Source: CAD feature listing. Evaluate the final solid. Frame: model axes, mm. Face numbers are marked on the shaded views. A direction names the side the tool comes from. Coordinates: 2 decimals unless noted, no trailing zeros. Write each loop counter-clockwise with the first axis right and the second up, starting at its lowest first coordinate (ties: lowest second). Pieces come first, ordered by that corner, then holes. Notation, with made-up numbers: M 21,-23.75 L 51,-23.75 A26 cw 51,8.25 Z; hole C 26.5,1.5 d2. An arc over 180 degrees is marked long. Write item = value, one per line. Start each with the question number.
1. Pin query (flat end, axial travel): pin 1 Ø0.9 at (y, z) = (8, -30) entering from -X; pin 2 Ø1.5 at (x, z) = (0, -37) entering from +Y; pin 3 Ø2 at (x, y) = (1.5, -9) entering from +Z; pin 4 Ø8 at (x, z) = (-14.5, -17.5) entering from +Y. Return the tip coordinate at first contact, or that it passes through.
2. Section query C-C (z = 19.5). Output: boundary loops of the cut face in (x, y), then the cut area to 3 significant figures.
3. Section query B-B (y = 2). Output: boundary loops of the cut face in (x, z), then the cut area to 3 significant figures.
4. Pull-direction query (X, two-part tool) for the marked faces 1, 2 and 3; classes: pulls with the +X half, pulls with the -X half, needs draft (parallel to the pull), parting line crosses it, or undercut.
5. Access query for the marked faces 4, 5 and 6. Directions: +Z, -Z, +X, -X, +Y, -Y. A direction counts if a zero-diameter tool reaches every point of the face in a straight line with its end or side. Return the directions, or none.
6. Section query D-D (z = -34.5). Output: boundary loops of the cut face in (x, y).
7. Line query: line 1 along Y through (x, z) = (0, 8) (3 decimals); line 2 along Y through (x, z) = (0, 5.8) (3 decimals); line 3 along Z through (x, y) = (9, -24). Output: solid intervals per line, ascending.
8. Section query A-A (x = 0). Output: boundary loops of the cut face in (y, z) (3 decimals), then the cut area to 3 significant figures.
Autodesk Inventor part; units mm, degrees
ref_plane "YZ Plane" through (0, 0, 0) normal (1, 0, 0) x (0, 1, 0)
ref_plane "XZ Plane" through (0, 0, 0) normal (0, 1, 0) x (-1, 0, 0)
ref_plane "XY Plane" through (0, 0, 0) normal (0, 0, 1) x (1, 0, 0)
sketch "Sketch1" plane through (0, 0, 0) normal (0, 0, 1) x (1, 0, 0)
  circle A0 centre (0, 0) radius 27.5 construction
  circle A1 centre (27.5, 0) radius 4.5
  circle A2 centre (13.75, 23.8157) radius 4.5
  circle A3 centre (-13.75, 23.8157) radius 4.5
  circle A4 centre (-27.5, 0) radius 4.5
  circle A5 centre (-13.75, -23.8157) radius 4.5
  circle A6 centre (13.75, -23.8157) radius 4.5
  circle A7 centre (0, 0) radius 35
  circle A8 centre (0, 0) radius 10
  circle A9 centre (0, 0) radius 12.5
  dimension "d0" = 55
  dimension "d1" = 9
  dimension "d4" = 360
  dimension "d6" = 70
  dimension "d11" = 20
  dimension "d19" = 2.5
extrude "Extrusion1" add sketch "Sketch1" along normal blind 10 contours A7 | A9
extrude "Extrusion2" add sketch "Sketch1" along normal blind 38 contours A1 | A2 | A3 | A4 | A5 | A6
sketch "Sketch3" plane through (0, 0, 10) normal (0, 0, 1) x (1, 0, 0)
  circle A0 centre (0, 0) radius 10
  circle A1 centre (0, 0) radius 13.025
  circle A2 centre (0, 0) radius 11.025
  dimension "d16" = 20
  dimension "d24" = 26.05
  dimension "d27" = 2
extrude "Extrusion4" add sketch "Sketch3" against normal blind 54 contours A0
extrude "Extrusion5" add sketch "Sketch1" against normal blind 2 contours A9
extrude "Extrusion7" cut sketch "Sketch3" against normal blind 5 contours A0 | A2
extrude "Extrusion8" cut sketch "Sketch3" against normal blind 3 contours A1
sketch "Sketch5" plane through (0, 0, -44) normal (0, 0, -1) x (-1, 0, 0)
  circle A0 centre (0, 0) radius 10
  circle A1 centre (0, 0) radius 9.95
  dimension "d30" = 0.05
extrude "Extrusion9" cut sketch "Sketch5" against normal up to surface (42 mm away)
sketch "Sketch6" plane through (0, 0, -44) normal (0, 0, -1) x (-1, 0, 0)
  circle A0 centre (0, 0) radius 9.95
  line L0 (-1.5, 7) -> (1.5, 7)
  line L1 (1.5, 7) -> (1.5, 12)
  line L2 (1.5, 12) -> (-1.5, 12)
  line L3 (-1.5, 12) -> (-1.5, 7)
  dimension "d35" = 1.5
  dimension "d36" = 1.5
  dimension "d38" = 7
extrude "Extrusion10" cut sketch "Sketch6" against normal blind 20 contours L1 L0 L3 A0 | A0 L3 L2 L1 picked at (0.1672, 7.9791)
properties part number "Output Shaft"
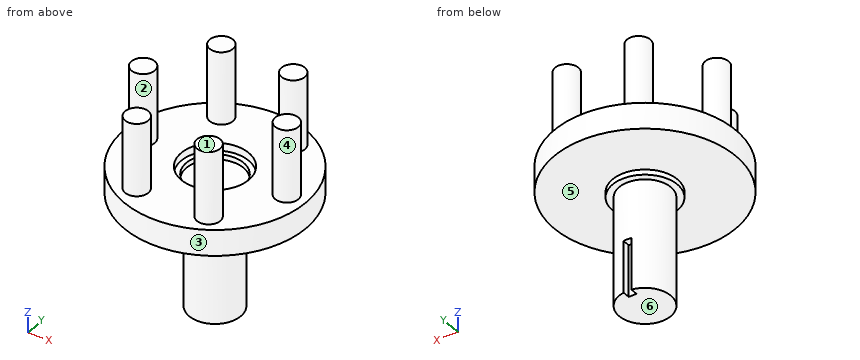
Results are:
q1.pin_1 = -6.48
q1.pin_2 = 7
q1.pin_3 = 5
q1.pin_4 = through
q2.outline = C -27.5,0 d9; C -13.75,-23.82 d9; C -13.75,23.82 d9; C 13.75,-23.82 d9; C 13.75,23.82 d9; C 27.5,0 d9
q2.area = 382 mm^2
q3.outline = M -34.94,0 L -12.34,0 L -12.34,-2 L -9.75,-2 L -9.75,-44 L 9.75,-44 L 9.75,-2 L 12.34,-2 L 12.34,0 L 34.94,0 L 34.94,10 L 31.53,10 L 31.53,38 L 23.47,38 L 23.47,10 L 12.87,10 L 12.87,7 L 10.84,7 L 10.84,5 L -10.84,5 L -10.84,7 L -12.87,7 L -12.87,10 L -23.47,10 L -23.47,38 L -31.53,38 L -31.53,10 L -34.94,10 Z
q3.area = 1,900 mm^2
q4.face_1 = needs draft
q4.face_2 = undercut
q4.face_3 = parting line crosses it
q5.face_4 = +Z
q5.face_5 = -Z
q5.face_6 = -Z, +X, -X, +Y, -Y
q6.outline = M -1.5,7 L -1.5,9.84 A9.95 ccw long 1.5,9.84 L 1.5,7 Z
q7.line_1 = -35 to -13.025, 13.025 to 35
q7.line_2 = -35 to -11.025, 11.025 to 35
q7.line_3 = 0 to 10
q8.outline = M -35,0 L -12.5,0 L -12.5,-2 L -9.95,-2 L -9.95,-44 L 7,-44 L 7,-24 L 9.95,-24 L 9.95,-2 L 12.5,-2 L 12.5,0 L 35,0 L 35,10 L 13.025,10 L 13.025,7 L 11.025,7 L 11.025,5 L -11.025,5 L -11.025,7 L -13.025,7 L -13.025,10 L -35,10 Z
q8.area = 1,400 mm^2
